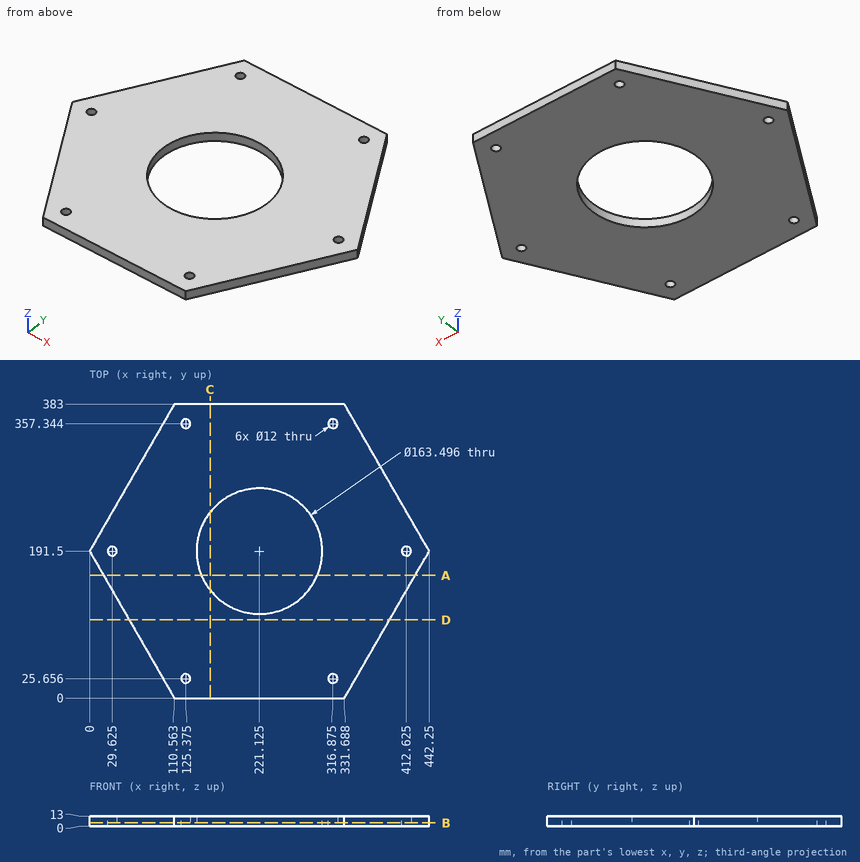
Could you check a few things on this drawing? It's one solid part, dimensions in mm from its lowest x, y, z. Round coordinates to 2 decimals unless told otherwise and drop trailing zeros. Loops run counter-clockwise (first coordinate to the right, second up) from the corner with the lowest first, then second, coordinate; pieces in that order, holes last. Notation, with made-up numbers: (4.25, 77) -> (22.25, 77) arc R17 ccw to (22.25, 84) -> close; hole circle Ø3 at (73.25, 78). An arc over 180 degrees is marked (long way). One line per item, written item: value. Start each with the question number.
1. If we section it at A-A, the plane y = 160: Write out the boundary of the cut face in (x, z).
2. If we section it at D-D, the plane y = 102: Write out the boundary of the cut face in (x, z).
3. If we section it at B-B, the plane z = 4.25: Give the number of separate pieces and of enclosed holes in the cut face, then the cut area to 3 significant figures.
4. If we section it at C-C, the plane x = 157: Write out the boundary of the cut face in (y, z), then the cut area to 3 significant figures.
5. For pin 1 (5 mm diameter, centred on x = 77, z = 11, fed in from -Y); pin 2 (1.5 mm diameter, centred on y = 182, z = 11, fed in from -X); pin 3 (6 mm diameter, centred on x = 220.5, z = 5, fed in from -Y); pin 4 (7 mm diameter, centred on x = 29.63, y = 191.5, fed in from -Z) (3 decimals), each with a flat end and sliding along its axis, tell me the tip position at first contact or that it passes through.
6. If I drill on probe 1 along X at (y, z) = (354, 12.5) (1 decimal); probe 2 along X at (y, z) = (221, 8.25) (1 decimal); probe 3 along Y at (x, z) = (251.5, 1) (1 decimal), over which ranges is the centre line in solid material (lowest first)?
Calculated:
1. outline: (18.19, 0) -> (145.69, 0) -> (145.69, 13) -> (18.19, 13) -> close; (296.56, 0) -> (424.06, 0) -> (424.06, 13) -> (296.56, 13) -> close
2. outline: (51.67, 0) -> (390.58, 0) -> (390.58, 13) -> (51.67, 13) -> close
3. separate pieces: 1
3. enclosed holes: 7
3. area: 105,000 mm²
4. outline: (0, 0) -> (140.8, 0) -> (140.8, 13) -> (0, 13) -> close; (242.2, 0) -> (383, 0) -> (383, 13) -> (242.2, 13) -> close
4. area: 3,660 mm²
5. pin 1: stops at y = 53.8
5. pin 2: stops at x = 5.05
5. pin 3: stops at y = 0
5. pin 4: passes through
6. probe 1: x = 93.8 to 120.4, 130.4 to 311.9, 321.9 to 348.4
6. probe 2: x = 17 to 144.9, 297.4 to 425.2
6. probe 3: y = 0 to 115.6, 267.4 to 383
